The model under review builds one solid part; all positions refer to its coordinate system, in mm. Round coordinates to 2 decimals unless told otherwise and drop trailing zeros. Write each loop counter-clockwise with the first axis right and the second up, starting at its lowest first coordinate (ties: lowest second). Pieces come first, ordered by that corner, then holes. Notation, with made-up numbers: (22.5, 17.25) -> (35.5, 17.25) arc R7 ccw to (35.5, 27.25) -> close; hole circle Ø10 at (31, -14). An arc over 180 degrees is marked (long way). Return JSON: item names as keys, results as strings. Group by question number.
1. Take a section at C-C, the plane y = 87. Write out the cut boundary in (x, z).
2. For line 1 along Y through (x, z) = (-227, 2.25); line 2 along Y through (x, z) = (-143, -9.75); line 3 along X through (y, z) = (-177, -8.25), list the stretches that pass through material, from the lowest coordinate up. Write a range as from..to.
3. Take a section at A-A, the plane x = -212. Write out the cut boundary in (y, z).
4. Clearance check with flat-ended pins moving along their axes: P1, Ø1.5, axis at x = 202, z = -2.5, coming from the +Y side; P2, Ø1, axis at x = 126, z = -9.5, coming from the +Y side; P3, Ø1, axis at x = 38.5, z = -10, coming from the +Y side. State where each tip first meets the part, or that it passes through.
5. Take a section at B-B, the plane y = -156. Write out the cut boundary in (x, z), then the cut area to 3 significant figures.
from build123d import *

# Parameters (mm, degrees)
F0_R     = 12.7
F4_DEPTH = 762


with BuildPart() as f2:
    # F2: sweep along a path in F1
    with BuildLine(Plane.XY) as f2_path:
        Line((0, 0), (0, 127))
        Line((0, 127), (215.9, 127))
        ThreePointArc((215.9, 127), (242.8407683632, 138.1592316368), (254, 165.1))
        ThreePointArc((254, 165.1), (242.8407683632, 192.0407683632), (215.9, 203.2))
        Line((215.9, 203.2), (-292.1, 203.2))
        ThreePointArc((-292.1, 203.2), (-319.0407683632, 192.0407683632), (-330.2, 165.1))
        ThreePointArc((-330.2, 165.1), (-319.0407683632, 138.1592316368), (-292.1, 127))
        Line((-292.1, 127), (-127, 127))
    # F0 (on Front) → F2 (sweep)
    with BuildSketch(Plane.XZ):
        Circle(F0_R)
    sweep(path=f2_path.line, transition=Transition.RIGHT)

    # F3 (on face) → F4 (join)
    with BuildSketch(Plane.XZ):
        Polygon((4.6947609848, 6.9345362704), (-4.1952390152, 6.9345362704), (-8.6402390152, -0.7644295692), (-4.1952390152, -8.4633954089), (4.6947609848, -8.4633954089), (9.1397609848, -0.7644295692), align=None)
    extrude(amount=F4_DEPTH)


solid = f2.part
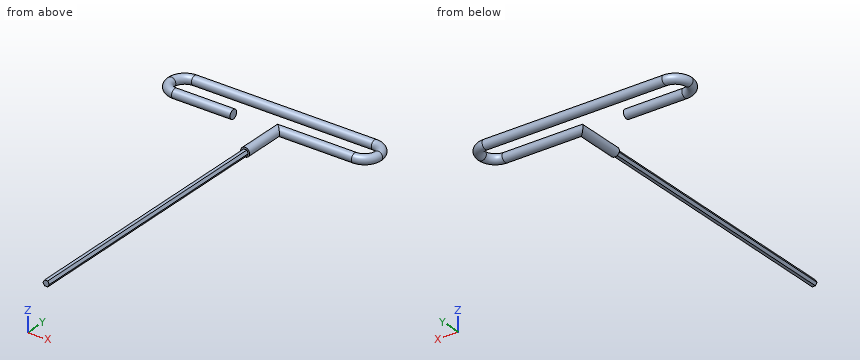
Output:
{
 "1": {"outline": "circle Ø25.4 at (0, 0)"},
 "2": {"line 1": "y = 114.5..139.5, 190.7..215.7", "line 2": "y = 118.86..135.14, 195.06..211.34", "line 3": "x = -4.32..4.82"},
 "3": {"outline": "circle Ø25.4 at (127, 0); circle Ø25.4 at (203.2, 0)"},
 "4": {"P1": "stops at y = 215.78", "P2": "stops at y = 212.16", "P3": "stops at y = 211.63"},
 "5": {"outline": "(-8.64, -0.76) -> (-4.2, -8.46) -> (4.69, -8.46) -> (9.14, -0.76) -> (4.69, 6.93) -> (-4.2, 6.93) -> close", "area": "205 mm^2"}
}
